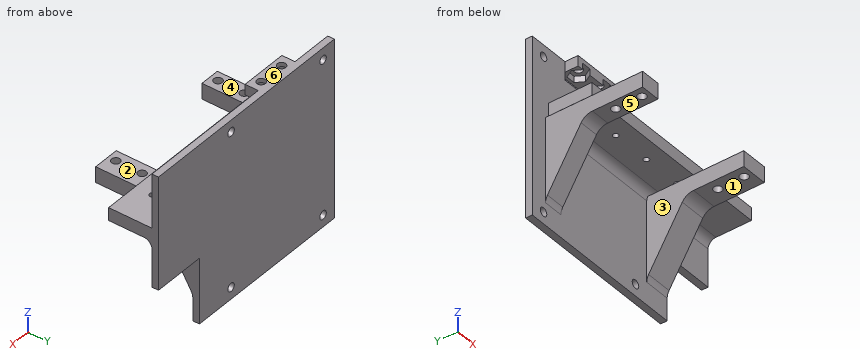
```python
from build123d import *

# Parameters (mm, degrees)
ORTHOGONAL_START                              = -15
ORTHOGONAL_CHASSIS_PLATE_PRIMARY_PROFILE_W    = 66
ORTHOGONAL_CHASSIS_PLATE_PRIMARY_PROFILE_H    = 4
ORTHOGONAL_CHASSIS_PLATE_PRIMARY_DEPTH        = 25.1
ORTHOGONAL_START_2                            = 10
ORTHOGONAL_CHASSIS_PLATE_GUIDE_SIDE_PROF_W    = 109
ORTHOGONAL_CHASSIS_PLATE_GUIDE_SIDE_PROF_H    = 4
ORTHOGONAL_CHASSIS_PLATE_GUIDE_SIDE_DEPTH     = 43
HORIZONTAL_START                              = 20
HORIZONTAL_SERVO_SEAT_UPRIGHTS_PROFILE_W      = 7.5
HORIZONTAL_SERVO_SEAT_UPRIGHTS_PROFILE_H      = 37.1
HORIZONTAL_SERVO_SEAT_UPRIGHTS_PROFILE_W_2    = 10
HORIZONTAL_SERVO_SEAT_UPRIGHTS_DEPTH          = 6
SIDE_START                                    = 27.5
SIDE_MOUNTING_FACE_FOR_MGN7_RAIL_PROFILE_W    = 100
SIDE_MOUNTING_FACE_FOR_MGN7_RAIL_PROFILE_H    = 16.6
SIDE_MOUNTING_FACE_FOR_MGN7_RAIL_DEPTH        = 4.9
HORIZONTAL_START_2                            = 49
HORIZONTAL_LIMIT_BRACKET_FOOT_SUPPORT_PR_W    = 18
HORIZONTAL_LIMIT_BRACKET_FOOT_SUPPORT_PR_H    = 5.1
HORIZONTAL_LIMIT_BRACKET_FOOT_SUPPORT_DEPTH   = 4
CHASSIS_START                                 = 28.9
CHASSIS_MOUNTING_HOLE_LAYOUT_45_X_41_2_R      = 1.6
CHASSIS_MOUNTING_HOLE_LAYOUT_45_X_41_MM_DEPTH = 4.2
SERVO_START                                   = 19.9
SERVO_MOUNT_50_X_10_MM_PITCH_PROFILE_R        = 1.6
SERVO_MOUNT_50_X_10_MM_PITCH_DEPTH            = 6.2
GUIDE_START                                   = 27.45
GUIDE_M2_MOUNTING_PILOTS_15_MM_PITCH_PRO_R    = 1.05
GUIDE_M2_MOUNTING_PILOTS_15_MM_PITCH_DEPTH    = 5.05
STOP_START                                    = 48.9
STOP_MOUNTING_TWO_M3_PILOTS_10_MM_PI_2_R      = 1.6
STOP_MOUNTING_TWO_M3_PILOTS_10_MM_PITCH_DEPTH = 4.2
FILLET_2_R                                    = 3
SKETCH_3_W                                    = 18
SKETCH_3_H                                    = 3
CUT_EXTRUDE_1_DEPTH                           = 2
CUT_EXTRUDE_2_DEPTH                           = 2.4
EXTRUDE_3_DEPTH                               = 7.5
EXTRUDE_4_DEPTH                               = 10
FILLET_3_R                                    = 5
SKETCH_7_W                                    = 109
SKETCH_7_H                                    = 1.5
CUT_EXTRUDE_3_DEPTH                           = 80
SKETCH_8_W                                    = 23
SKETCH_8_H                                    = 43
CUT_EXTRUDE_4_DEPTH                           = 30


with BuildPart() as part:
    # Orthogonal chassis plate primary profile → Orthogonal chassis plate primary (new body)
    with BuildSketch(Plane.XY.offset(ORTHOGONAL_START)):
        with Locations((8, 31)):
            Rectangle(ORTHOGONAL_CHASSIS_PLATE_PRIMARY_PROFILE_W, ORTHOGONAL_CHASSIS_PLATE_PRIMARY_PROFILE_H)
    extrude(amount=ORTHOGONAL_CHASSIS_PLATE_PRIMARY_DEPTH)

    # Orthogonal chassis plate guide side profile → Orthogonal chassis plate guide side (add)
    with BuildSketch(Plane.XY.offset(ORTHOGONAL_START_2)):
        with Locations((29.5, 31)):
            Rectangle(ORTHOGONAL_CHASSIS_PLATE_GUIDE_SIDE_PROF_W, ORTHOGONAL_CHASSIS_PLATE_GUIDE_SIDE_PROF_H)
    extrude(amount=ORTHOGONAL_CHASSIS_PLATE_GUIDE_SIDE_DEPTH)

    # Horizontal servo seat uprights profile → Horizontal servo seat uprights (add)
    with BuildSketch(Plane.XY.offset(HORIZONTAL_START)):
        with Locations((-14.75, 10.55)):
            Rectangle(HORIZONTAL_SERVO_SEAT_UPRIGHTS_PROFILE_W, HORIZONTAL_SERVO_SEAT_UPRIGHTS_PROFILE_H)
        with Locations((36, 10.55)):
            Rectangle(HORIZONTAL_SERVO_SEAT_UPRIGHTS_PROFILE_W_2, HORIZONTAL_SERVO_SEAT_UPRIGHTS_PROFILE_H)
    extrude(amount=HORIZONTAL_SERVO_SEAT_UPRIGHTS_DEPTH)

    # Side mounting face for MGN7 rail profile → Side mounting face for MGN7 rail (add)
    with BuildSketch(Plane.XY.offset(SIDE_START)):
        with Locations((33, 20.8)):
            Rectangle(SIDE_MOUNTING_FACE_FOR_MGN7_RAIL_PROFILE_W, SIDE_MOUNTING_FACE_FOR_MGN7_RAIL_PROFILE_H)
    extrude(amount=SIDE_MOUNTING_FACE_FOR_MGN7_RAIL_DEPTH)

    # Horizontal limit bracket foot support profile → Horizontal limit bracket foot support (add)
    with BuildSketch(Plane.XY.offset(HORIZONTAL_START_2)):
        with Locations((0, 26.55)):
            Rectangle(HORIZONTAL_LIMIT_BRACKET_FOOT_SUPPORT_PR_W, HORIZONTAL_LIMIT_BRACKET_FOOT_SUPPORT_PR_H)
    extrude(amount=HORIZONTAL_LIMIT_BRACKET_FOOT_SUPPORT_DEPTH)

    # Chassis mounting hole layout 45 x 41 2 → Chassis mounting hole layout 45 x 41 mm (cut)
    with BuildSketch(Plane(origin=(0, 0, 0), x_dir=(1, 0, 0), z_dir=(0, 1, 0)).offset(CHASSIS_START)):
        with Locations(Location((-19.5, 10.5, 0), (0, 0, 90))):
            Circle(CHASSIS_MOUNTING_HOLE_LAYOUT_45_X_41_2_R)
        with Locations(Location((-19.5, -48.5, 0), (0, 0, 90))):
            Circle(CHASSIS_MOUNTING_HOLE_LAYOUT_45_X_41_2_R)
        with Locations(Location((25.5, 10.5, 0), (0, 0, 90))):
            Circle(CHASSIS_MOUNTING_HOLE_LAYOUT_45_X_41_2_R)
        with Locations(Location((25.5, -48.5, 0), (0, 0, 90))):
            Circle(CHASSIS_MOUNTING_HOLE_LAYOUT_45_X_41_2_R)
        with Locations(Location((70.5, -48.5, 0), (0, 0, 90))):
            Circle(CHASSIS_MOUNTING_HOLE_LAYOUT_45_X_41_2_R)
    extrude(amount=CHASSIS_MOUNTING_HOLE_LAYOUT_45_X_41_MM_DEPTH, mode=Mode.SUBTRACT)

    # Servo mount 50 x 10 mm pitch profile → Servo mount 50 x 10 mm pitch (cut)
    with BuildSketch(Plane.XY.offset(SERVO_START)):
        with Locations(Location((-15, -5, 0), (0, 0, 180))):
            Circle(SERVO_MOUNT_50_X_10_MM_PITCH_PROFILE_R)
        with Locations(Location((-15, 5, 0), (0, 0, 180))):
            Circle(SERVO_MOUNT_50_X_10_MM_PITCH_PROFILE_R)
        with Locations(Location((35, -5, 0), (0, 0, 180))):
            Circle(SERVO_MOUNT_50_X_10_MM_PITCH_PROFILE_R)
        with Locations(Location((35, 5, 0), (0, 0, 180))):
            Circle(SERVO_MOUNT_50_X_10_MM_PITCH_PROFILE_R)
    extrude(amount=SERVO_MOUNT_50_X_10_MM_PITCH_DEPTH, mode=Mode.SUBTRACT)

    # Guide M2 mounting pilots 15 mm pitch profile → Guide M2 mounting pilots 15 mm pitch (cut)
    with BuildSketch(Plane.XY.offset(GUIDE_START)):
        with Locations((-12, 19)):
            Circle(GUIDE_M2_MOUNTING_PILOTS_15_MM_PITCH_PRO_R)
        with Locations((3, 19)):
            Circle(GUIDE_M2_MOUNTING_PILOTS_15_MM_PITCH_PRO_R)
        with Locations((18, 19)):
            Circle(GUIDE_M2_MOUNTING_PILOTS_15_MM_PITCH_PRO_R)
        with Locations((33, 19)):
            Circle(GUIDE_M2_MOUNTING_PILOTS_15_MM_PITCH_PRO_R)
        with Locations((48, 19)):
            Circle(GUIDE_M2_MOUNTING_PILOTS_15_MM_PITCH_PRO_R)
        with Locations((63, 19)):
            Circle(GUIDE_M2_MOUNTING_PILOTS_15_MM_PITCH_PRO_R)
        with Locations((78, 19)):
            Circle(GUIDE_M2_MOUNTING_PILOTS_15_MM_PITCH_PRO_R)
    extrude(amount=GUIDE_M2_MOUNTING_PILOTS_15_MM_PITCH_DEPTH, mode=Mode.SUBTRACT)

    # Stop mounting two M3 pilots 10 mm pi 2 → Stop mounting two M3 pilots 10 mm pitch (cut)
    with BuildSketch(Plane.XY.offset(STOP_START)):
        with Locations((-5, 27)):
            Circle(STOP_MOUNTING_TWO_M3_PILOTS_10_MM_PI_2_R)
        with Locations((5, 27)):
            Circle(STOP_MOUNTING_TWO_M3_PILOTS_10_MM_PI_2_R)
    extrude(amount=STOP_MOUNTING_TWO_M3_PILOTS_10_MM_PITCH_DEPTH, mode=Mode.SUBTRACT)

    # 圆角2
    # the kernel refuses this fillet: 3 mm, written as the material it adds along each edge
    with BuildSketch(Plane(origin=(-17, 29, 27.5), x_dir=(0, 0, -1), z_dir=(1, 0, 0))) as fillet_2_piece_1:
        with BuildLine():
            CenterArc((FILLET_2_R, -FILLET_2_R), FILLET_2_R, 90, 90)
            Line((0, -FILLET_2_R), (0, 0))
            Line((0, 0), (FILLET_2_R, 0))
        make_face()
    extrude(amount=100)

    # 草图3 → 切除-拉伸1 (cut)
    with BuildSketch(Plane(origin=(0, 29, 0), x_dir=(-1, 0, 0), z_dir=(0, -1, 0))):
        with Locations((0, -47.5)):
            Rectangle(SKETCH_3_W, SKETCH_3_H)
    extrude(amount=-CUT_EXTRUDE_1_DEPTH, mode=Mode.SUBTRACT)

    # 草图4 → 切除-拉伸2 (cut)
    with BuildSketch(Plane(origin=(0, 0, 49), x_dir=(-1, 0, 0), z_dir=(0, 0, -1))):
        Polygon((-3.267949192, 30), (-6.732050808, 30), (-8.464101615, 27), (-6.732050808, 24), (-3.267949192, 24), (-1.535898385, 27), align=None)
        Polygon((6.732050808, 30), (3.267949192, 30), (1.535898385, 27), (3.267949192, 24), (6.732050808, 24), (8.464101615, 27), align=None)
    extrude(amount=-CUT_EXTRUDE_2_DEPTH, mode=Mode.SUBTRACT)

    # 草图5 → 凸台-拉伸3 (add)
    with BuildSketch(Plane(origin=(-11, 0, 0), x_dir=(0, 0, -1), z_dir=(1, 0, 0))):
        Polygon((-20, 29), (5, 29), (-20, 14), align=None)
    extrude(amount=-EXTRUDE_3_DEPTH)

    # 草图6 → 凸台-拉伸4 (add)
    with BuildSketch(Plane.ZY.offset(-31)):
        Polygon((20, 29), (-5, 29), (20, 14), align=None)
    extrude(amount=-EXTRUDE_4_DEPTH)

    # 圆角3
    fillet_3_edges = [part.edges().sort_by_distance(p)[0] for p in [
        (-14.75, 14, 20),
        (-14.75, 29, -5),
        (36, 14, 20),
        (36, 29, -5),
    ]]
    fillet(fillet_3_edges, radius=FILLET_3_R)

    # 草图7 → 切除-拉伸3 (cut)
    with BuildSketch(Plane.XY.offset(53)):
        with Locations((29.5, 32.25)):
            Rectangle(SKETCH_7_W, SKETCH_7_H)
    extrude(amount=-CUT_EXTRUDE_3_DEPTH, mode=Mode.SUBTRACT)

    # 草图8 → 切除-拉伸4 (cut)
    with BuildSketch(Plane(origin=(0, 31.5, 0), x_dir=(1, 0, 0), z_dir=(0, 1, 0))):
        with Locations((72.5, -31.5)):
            Rectangle(SKETCH_8_W, SKETCH_8_H)
    extrude(amount=-CUT_EXTRUDE_4_DEPTH, mode=Mode.SUBTRACT)


solid = part.part
```
Check sheet for the modelled part. Datum: model origin and axes. Units: mm. Face numbers are marked on the shaded views. A direction names the side the tool comes from. Round coordinates to 2 decimals unless told otherwise and drop trailing zeros. Order: outer loops, then holes, each group sorted by start corner. A loop starts at its lowest first (then second) coordinate and runs counter-clockwise, first axis right, second up.
1) Section check D-D (x = 55.5). Record the boundary of the cut face in (y, z), and give its area (3 significant figures).
2) Section check C-C (x = 5). Record the boundary of the cut face in (y, z).
3) Go/stop test with flat-tipped pins: pin 1 Ø3 at (x, z) = (-19.5, 48.5) entering from +Y; pin 2 Ø1.5 at (x, z) = (30.5, 30) entering from -Y; pin 3 Ø6 at (x, y) = (46, 24.5) entering from +Z; pin 4 Ø4 at (x, y) = (-15, 5) entering from +Z. Record where each tip stops, or that it passes through.
4) Section check A-A (y = -1). Record the boundary of the cut face in (x, z), and give its area (3 significant figures).
5) Scan lines: line 1 (X direction, y = 29.5, z = 48.5); line 2 (Y direction, x = 35, z = 23.3); line 3 (X direction, y = 3, z = 22). Record each from-to range of solid material in increasing order.
6) Mould release check, pull along Z, two halves, no side actions. Record for the marked faces 4, 5 and 6: +Z half, -Z half, draft (parallel to the pull), parting line (faces both ways), or undercut.
7) Section check B-B (x = -15). Record the boundary of the cut face in (y, z), and give its area (3 significant figures).
8) Tool access check on the marked faces 1, 2 and 3. Record the directions out of +Z, -Z, +X, -X, +Y, -Y that give a thin tool (end or side, any length) a straight path to the whole face; none if there is none.
Result:
1. outline: (12.5, 27.5) - (26, 27.5) arc R3 cw to (29, 24.5) - (29, 10) - (31.5, 10) - (31.5, 53) - (29, 53) - (29, 32.4) - (12.5, 32.4) - close
1. area: 190 mm2
2. outline: (12.5, 27.5) - (26, 27.5) arc R3 cw to (29, 24.5) - (29, -15) - (31.5, -15) - (31.5, 53) - (28.6, 53) - (28.6, 51.4) - (30, 51.4) - (30, 49) - (31, 49) - (31, 46) - (29, 46) - (29, 32.4) - (12.5, 32.4) - close; (24, 51.4) - (25.4, 51.4) - (25.4, 53) - (24, 53) - close
3. pin 1: passes through
3. pin 2: stops at y = 12.5
3. pin 3: stops at z = 32.4
3. pin 4: stops at z = 26
4. outline: (-18.5, 20) - (-11, 20) - (-11, 26) - (-18.5, 26) - close; (31, 20) - (41, 20) - (41, 26) - (31, 26) - close
4. area: 105 mm2
5. line 1: x = -25 to -21.1, -17.9 to -9, 9 to 23.9, 27.1 to 61
5. line 2: y = -8 to -6.6, -3.4 to 3.4, 6.6 to 31.5
5. line 3: x = -18.5 to -11, 31 to 41
6. face 4: undercut
6. face 5: -Z half
6. face 6: +Z half
7. outline: (-8, 20) - (-6.6, 20) - (-6.6, 26) - (-8, 26) - close; (-3.4, 20) - (3.4, 20) - (3.4, 26) - (-3.4, 26) - close; (6.6, 20) - (11.17, 20) arc R5 cw to (15.46, 17.57) - (28.29, -3.81) arc R5 cw to (29, -6.38) - (29, -15) - (31.5, -15) - (31.5, 53) - (29, 53) - (29, 32.4) - (12.5, 32.4) - (12.5, 27.5) - (26, 27.5) arc R3 cw to (28.6, 26) - (6.6, 26) - close
7. area: 625 mm2
8. face 1: -Z, +X, -X, -Y
8. face 2: +X, -X, -Y
8. face 3: -Z, -Y
